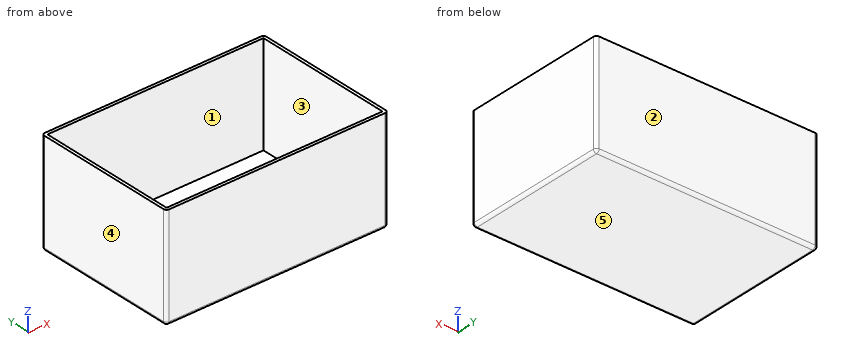
```python
from build123d import *

# Parameters (mm, degrees)
SKETCH_W    = 71
SKETCH_H    = 46
PAD_DEPTH   = 33
THICKNESS_T = 1


with BuildPart() as part:
    # Sketch → Pad (new body)
    with BuildSketch(Plane.XY):
        with Locations((35.5, 23)):
            Rectangle(SKETCH_W, SKETCH_H)
    extrude(amount=PAD_DEPTH)

    # Thickness
    thickness_openings = [part.faces().sort_by_distance(p)[0] for p in [
        (35.5, 23, 33),
    ]]
    offset(amount=THICKNESS_T, openings=thickness_openings)


solid = part.part
```
For this review, take the finished solid that the model builds, in its own axes (mm). Face numbers are marked on the shaded views. A direction names the side the tool comes from. Give positions to 0.01 mm unless a question says otherwise; leave off trailing zeros. Write each loop counter-clockwise with the first axis right and the second up, starting at its lowest first coordinate (ties: lowest second). Pieces come first, ordered by that corner, then holes. Notation, with made-up numbers: M 4,-10.5 L 57,-10.5 A17 cw 57,-2.5 Z; hole C 33,59 d9. An arc over 180 degrees is marked long. Answer as CSV lines item,"result".
1. Consider section B-B, the plane x = 48.5. Write out the cut boundary in (y, z), then the cut area to 3 significant figures.
Findings:
outline,"M -1,0 A1 ccw 0,-1 L 46,-1 A1 ccw 47,0 L 47,33 L 46,33 L 46,0 L 0,0 L 0,33 L -1,33 Z"
area,"114 mm2"
2. For pin 1 (12 mm diameter, centred on x = 9.5, y = 38, fed in from +Z), flat-tipped, find the tip position at first contact; note if it passes through.
Findings:
pin 1,"stops at z = 0"
3. Wall thickness on line 1 (Y direction, x = 59.5, z = 22.5); line 2 (X direction, y = 39.5, z = 20); line 3 (Z direction, x = 30, y = 14.5): over which ranges is each line inside the solid? List them lowest first.
Findings:
line 1,"y = -1 to 0, 46 to 47"
line 2,"x = -1 to 0, 71 to 72"
line 3,"z = -1 to 0"
4. For the marked faces 1 and 2, list the 3-axis set-ups (+Z, -Z, +X, -X, +Y, -Y) from which the entire face can be reached by the end or side of a thin tool; tool diameter is ignored.
Findings:
face 1,"+Z"
face 2,"+Z, -Z, +X, -X, +Y"
5. Draft analysis for pull direction X (two halves, no side actions). For the marked faces 3, 4 and 5, state which applies: +X half, -X half, draft (parallel to the pull), parting line (faces both ways), or undercut.
Findings:
face 3,"undercut"
face 4,"-X half"
face 5,"draft"
6. Consider section C-C, the plane y = 9.5. Write out the cut boundary in (x, z).
Findings:
outline,"M -1,0 A1 ccw 0,-1 L 71,-1 A1 ccw 72,0 L 72,33 L 71,33 L 71,0 L 0,0 L 0,33 L -1,33 Z"
7. Consider section A-A, the plane z = 20.5. Write out the cut boundary in (x, y), then the cut area to 3 significant figures.
Findings:
outline,"M -1,0 A1 ccw 0,-1 L 71,-1 A1 ccw 72,0 L 72,46 A1 ccw 71,47 L 0,47 A1 ccw -1,46 Z; hole M 0,0 L 71,0 L 71,46 L 0,46 Z"
area,"237 mm2"
